from build123d import *

# Parameters (mm, degrees)
SALIENTE_EXTRUIR1_DEPTH = 4
CROQUIS3_R              = 1.75
CORTAR_EXTRUIR1_DEPTH   = 54.742441329
REDONDEO8_R             = 4
REDONDEO9_R             = 3
SALIENTE_EXTRUIR2_START = 6
CROQUIS4_R              = 4
CROQUIS4_R_2            = 1.75
SALIENTE_EXTRUIR2_DEPTH = 6
CROQUIS5_R              = 3.1
CORTAR_EXTRUIR2_DEPTH   = 3.2


with BuildPart() as part:
    # Croquis2 → Saliente-Extruir1 (new, symmetric)
    with BuildSketch(Plane(origin=(0, 0, 0), x_dir=(1, 0, 0), z_dir=(0, 1, 0))):
        Polygon((27.5, -23), (27.5, -15), (4, -15), (4, 15), (27.5, 15), (27.5, 23), (-27.5, 23), (-27.5, 15), (-4, 15), (-4, -15), (-27.5, -15), (-27.5, -23), align=None)
    extrude(amount=SALIENTE_EXTRUIR1_DEPTH, both=True)

    # Croquis3 → Cortar-Extruir1 (cut, through all)
    with BuildSketch(Plane.XY.offset(23)):
        with Locations((23.5, 0)):
            Circle(CROQUIS3_R)
        with Locations((-23.5, 0)):
            Circle(CROQUIS3_R)
    extrude(amount=-CORTAR_EXTRUIR1_DEPTH, mode=Mode.SUBTRACT)

    # Redondeo8
    redondeo8_edges = [part.edges().sort_by_distance(p)[0] for p in [
        (27.5, -4, -19),
        (27.5, 4, -19),
        (27.5, -4, 19),
        (27.5, 4, 19),
        (-27.5, -4, -19),
        (-27.5, 4, -19),
        (-27.5, -4, 19),
        (-27.5, 4, 19),
    ]]
    fillet(redondeo8_edges, radius=REDONDEO8_R - 0.0001)  # a hair under: the kernel refuses the full size

    # Redondeo9
    redondeo9_edges = [part.edges().sort_by_distance(p)[0] for p in [
        (4, 0, -15),
        (4, 0, 15),
        (-4, 0, 15),
        (-4, 0, -15),
    ]]
    fillet(redondeo9_edges, radius=REDONDEO9_R)

    # Croquis4 → Saliente-Extruir2 (add)
    with BuildSketch(Plane.XY.offset(23).offset(SALIENTE_EXTRUIR2_START)):
        with Locations((23.5, 0)):
            Circle(CROQUIS4_R)
        with Locations((23.5, 0)):
            Circle(CROQUIS4_R_2, mode=Mode.SUBTRACT)
    extrude(amount=-SALIENTE_EXTRUIR2_DEPTH)

    # Croquis5 → Cortar-Extruir2 (cut)
    with BuildSketch(Plane(origin=(0, 0, -23), x_dir=(-1, 0, 0), z_dir=(0, 0, -1))):
        with Locations((-23.5, 0)):
            Circle(CROQUIS5_R)
    extrude(amount=-CORTAR_EXTRUIR2_DEPTH, mode=Mode.SUBTRACT)


solid = part.part
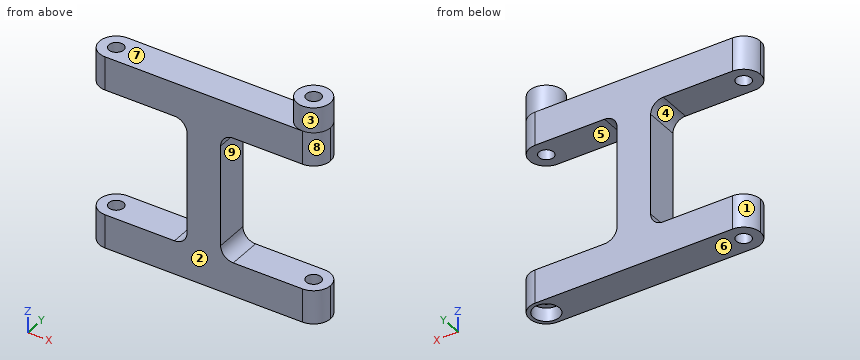
Source: CAD feature listing. Evaluate the final solid. Frame: model axes, mm. Face numbers are marked on the shaded views. A direction names the side the tool comes from. Coordinates: 2 decimals unless noted, no trailing zeros. Loops run counter-clockwise (first coordinate to the right, second up) from the corner with the lowest first, then second, coordinate; pieces in that order, holes last. Notation, with made-up numbers: (49, 37.25) - (70, 37.25) arc R14 cw to (70, 63.25) - close; hole circle Ø3 at (44.25, 53). An arc over 180 degrees is marked (long way). Return JSON: item names as keys, results as strings.
Q1. Section A-A, the plane x = 13.5. Return loops of the section in (y, z), plus the area to 3 significant figures.
Results:
{"outline": "(-4, -23) - (4, -23) - (4, -15) - (-4, -15) - close; (-4, 15) - (4, 15) - (4, 23) - (-4, 23) - close", "area": "128 mm2"}
Q2. Access query for the marked faces 1, 2, 3, 4 and 5. Directions: +Z, -Z, +X, -X, +Y, -Y. A direction counts if a zero-diameter tool reaches every point of the face in a straight line with its end or side. Return the directions, or none.
Results:
{"face 1": "+Z, -Z, -X, +Y", "face 2": "+Z, -Z, +X, -X, -Y", "face 3": "+Z", "face 4": "-X, +Y, -Y", "face 5": "+X, +Y, -Y"}
Q3. Section B-B, the plane z = -2.5. Return loops of the section in (x, y), plus the area to 3 significant figures.
Results:
{"outline": "(-4, -4) - (4, -4) - (4, 4) - (-4, 4) - close", "area": "64.0 mm2"}
Q4. Material intervals for line 1 along Z through (x, y) = (18, 1.75); line 2 along Y through (x, z) = (23.5, 25.5); line 3 along Z through (x, y) = (23, 3), sorted ascending.
Results:
{"line 1": "-23 to -15, 15 to 23", "line 2": "-4 to -1.75, 1.75 to 4", "line 3": "-19.8 to -15, 15 to 29"}
Q5. Section C-C, the plane y = -0.75. Give the number of separate pieces and of enclosed holes in the cut face, plus the area to 3 significant figures.
Results:
{"separate pieces": "5", "enclosed holes": "0", "area": "1,040 mm2"}
Q6. Contact query for flat-ended pins moving along their axis: P1, Ø3, axis at x = 23.5, y = 1, coming from the -Z side; P2, Ø1.5, axis at y = -2.5, z = 11.5, coming from the +X side; P3, Ø4, axis at y = 1.5, z = 9.5, coming from the -X side. Output: stop coordinate, or through.
Results:
{"P1": "z = -19.8", "P2": "x = 4.01", "P3": "x = -4"}
Q7. Mould query, pull axis Z, two halves, no side actions, for the marked faces 6, 7, 8 and 9. Classes: released by +Z, released by -Z, zero draft, split by the parting line, or undercut.
Results:
{"face 6": "released by -Z", "face 7": "released by +Z", "face 8": "zero draft", "face 9": "undercut"}
